```python
from build123d import *

# Parameters (mm, degrees)
SKETCH1_W           = 51.6
SKETCH1_H           = 38.8
BOSS_EXTRUDE1_DEPTH = 20.5
SKETCH2_W           = 51.6
SKETCH2_H           = 27.8
BOSS_EXTRUDE2_DEPTH = 14
SKETCH3_W           = 34.5
SKETCH3_H           = 38.8
BOSS_EXTRUDE3_DEPTH = 18
SKETCH4_W           = 0.75
SKETCH4_H           = 10
SKETCH4_W_2         = 1
BOSS_EXTRUDE4_DEPTH = 0.1
CHAMFER1_SIZE       = 2.5
CHAMFER2_SIZE       = 4.5


with BuildPart() as part:
    # Sketch1 → Boss-Extrude1 (new body)
    with BuildSketch(Plane.XY):
        Rectangle(SKETCH1_W, SKETCH1_H)
    extrude(amount=BOSS_EXTRUDE1_DEPTH)

    # Sketch2 → Boss-Extrude2 (add)
    with BuildSketch(Plane.XY.offset(20.5)):
        Rectangle(SKETCH2_W, SKETCH2_H)
    extrude(amount=BOSS_EXTRUDE2_DEPTH)

    # Sketch3 → Boss-Extrude3 (add)
    with BuildSketch(Plane.XY.offset(20.5)):
        with Locations((-1.95, 0)):
            Rectangle(SKETCH3_W, SKETCH3_H)
    extrude(amount=BOSS_EXTRUDE3_DEPTH)

    # Sketch4 → Boss-Extrude4 (add)
    with BuildSketch(Plane.XZ.offset(19.4)):
        with Locations((-13.325, 20)):
            Rectangle(SKETCH4_W, SKETCH4_H)
        with Locations((-11.075, 20)):
            Rectangle(SKETCH4_W, SKETCH4_H)
        with Locations((-8.825, 20)):
            Rectangle(SKETCH4_W, SKETCH4_H)
        with Locations((-6.575, 20)):
            Rectangle(SKETCH4_W, SKETCH4_H)
        with Locations((-4.325, 20)):
            Rectangle(SKETCH4_W, SKETCH4_H)
        with Locations((-2.075, 20)):
            Rectangle(SKETCH4_W, SKETCH4_H)
        with Locations((0.175, 20)):
            Rectangle(SKETCH4_W, SKETCH4_H)
        with Locations((2.425, 20)):
            Rectangle(SKETCH4_W, SKETCH4_H)
        with Locations((4.675, 20)):
            Rectangle(SKETCH4_W, SKETCH4_H)
        with Locations((6.925, 20)):
            Rectangle(SKETCH4_W, SKETCH4_H)
        with Locations((9.3, 20)):
            Rectangle(SKETCH4_W_2, SKETCH4_H)
    boss_extrude4 = extrude(amount=BOSS_EXTRUDE4_DEPTH)

    # Mirror1: Boss-Extrude4 across plane
    add(boss_extrude4.mirror(Plane.ZX))

    # Chamfer1
    chamfer1_edges = [part.edges().sort_by_distance(p)[0] for p in [
        (25.8, -19.4, 10.25),
        (-25.8, 19.4, 10.25),
        (-25.8, -19.4, 10.25),
        (25.8, 19.4, 10.25),
    ]]
    chamfer(chamfer1_edges, length=CHAMFER1_SIZE)

    # Chamfer2
    chamfer2_edges = [part.edges().sort_by_distance(p)[0] for p in [
        (-19.2, -19.4, 29.5),
        (15.3, -19.4, 29.5),
        (-19.2, 19.4, 29.5),
        (15.3, 19.4, 29.5),
    ]]
    chamfer(chamfer2_edges, length=CHAMFER2_SIZE)


solid = part.part
```
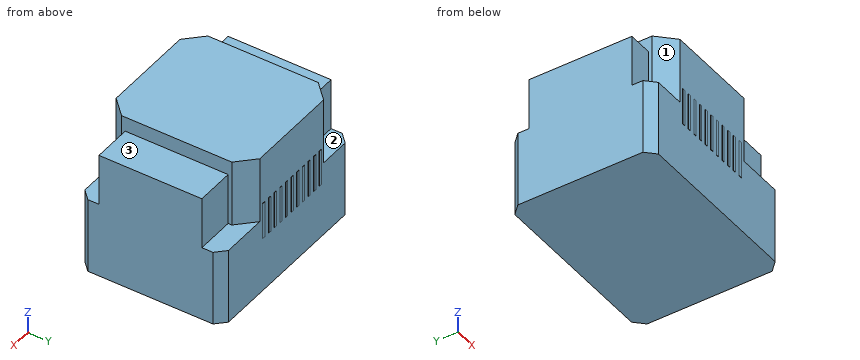
The listing builds one solid part. Answer for the finished solid, in the listing's coordinates (mm). Face numbers are marked on the shaded views. A direction names the side the tool comes from. Round coordinates to 2 decimals unless told otherwise and drop trailing zeros. Loops run counter-clockwise (first coordinate to the right, second up) from the corner with the lowest first, then second, coordinate; pieces in that order, holes last. Notation, with made-up numbers: (33, 61) -> (82, 61) arc R25 cw to (82, 84) -> close; hole circle Ø8 at (84.5, 43). An arc over 180 degrees is marked (long way). Use one line per item in the form item = value.
1. A tool of negligible diameter and unlimited length cuts with its end or side. For the marked faces 1, 2 and 3, from which of +Z, -Z, +X, -X, +Y, -Y can it reach the whole face along a straight path? Write none if from no direction.
Answer key:
face_1 = +Z, -X, -Y
face_2 = +Z, -X, +Y
face_3 = +Z, +X, +Y, -Y
2. Find the intervals of material crossed by probe 1 along Y at (x, z) = (-10, 5); probe 2 along X at (y, z) = (-7.5, 35); probe 3 along Z at (x, y) = (19, 16), in increasing order. Write a range as [from, to].
Answer key:
probe_1 = [-19.4, 19.4]
probe_2 = [-19.2, 15.3]
probe_3 = [0, 20.5]
3. Flat-ended cylindrical pins translate along their axes: pin 1 Ø4.5 at (x, y) = (17, -17.5) entering from +Z; pin 2 Ø6 at (x, z) = (0, 10.5) entering from -Y; pin 3 Ø12 at (x, z) = (-16, 4.5) entering from +Y. Find the tip coordinate at first contact, or state that the pin passes through.
Answer key:
pin_1 = 20.5
pin_2 = -19.4
pin_3 = 19.4
4. The part is cut by section B-B on y = 11. Determine the outline of the cut face in (x, z), and give its area (3 significant figures).
Answer key:
outline = (-25.8, 0) -> (25.8, 0) -> (25.8, 34.5) -> (15.3, 34.5) -> (15.3, 38.5) -> (-19.2, 38.5) -> (-19.2, 34.5) -> (-25.8, 34.5) -> close
area = 1,920 mm²
5. The part is cut by section A-A on z = 29. Determine the outline of the cut face in (x, y), and give its area (3 significant figures).
Answer key:
outline = (-25.8, -13.9) -> (-19.2, -13.9) -> (-19.2, -14.9) -> (-14.7, -19.4) -> (10.8, -19.4) -> (15.3, -14.9) -> (15.3, -13.9) -> (25.8, -13.9) -> (25.8, 13.9) -> (15.3, 13.9) -> (15.3, 14.9) -> (10.8, 19.4) -> (-14.7, 19.4) -> (-19.2, 14.9) -> (-19.2, 13.9) -> (-25.8, 13.9) -> close
area = 1,770 mm²
6. The part is cut by section C-C on x = 21. Determine the outline of the cut face in (y, z).
Answer key:
outline = (-19.4, 0) -> (19.4, 0) -> (19.4, 20.5) -> (13.9, 20.5) -> (13.9, 34.5) -> (-13.9, 34.5) -> (-13.9, 20.5) -> (-19.4, 20.5) -> close
